Here's how the part is built. I have some questions about the finished solid (model axes, mm). A direction names the side the tool comes from. Coordinates: 2 decimals unless noted, no trailing zeros. Write each loop counter-clockwise with the first axis right and the second up, starting at its lowest first coordinate (ties: lowest second). Pieces come first, ordered by that corner, then holes. Notation, with made-up numbers: (34.25, -9) -> (50.25, -9) arc R22 cw to (50.25, 8) -> close; hole circle Ø3 at (57.25, 27). An arc over 180 degrees is marked (long way). Put each result on its own line as item: value.
Autodesk Inventor part; units mm, degrees
ref_plane "Work Plane1" through (0, -11, 0) normal (0, 1, 0) x (-1, 0, 0)
ref_plane "Work Plane2" through (9.5263, 5.5, -10) normal (0.866, 0.5, 0) x (-0.5, 0.866, 0)
ref_plane "Work Plane3" through (-9.5263, 5.5, -10) normal (-0.866, 0.5, 0) x (-0.5, -0.866, 0)
sketch "Sketch1" plane through (0, 0, 0) normal (0, 0, 1) x (1, 0, 0)
  circle A0 centre (0, 0) radius 35
  dimension "d0" = 70
extrude "Extrusion1" add sketch "Sketch1" along normal blind 7
sketch "Sketch2" plane through (0, 0, 7) normal (0, 0, 1) x (1, 0, 0)
  circle A0 centre (0, 0) radius 35
  circle A1 centre (0, 0) radius 23 construction
  line L0 (0, 0) -> (0, 23) construction
  point P0 (-16.2635, 16.2635)
  point P1 (-23, 0)
  point P2 (-16.2635, -16.2635)
  point P3 (0, -23)
  point P4 (16.2635, -16.2635)
  point P5 (23, 0)
  point P6 (16.2635, 16.2635)
  dimension "d3" = 46
  dimension "d6" = 360
hole "Hole1" at (0, 23, 7) at (-16.2635, 16.2635, 7) at (-23, 0, 7) at (-16.2635, -16.2635, 7) at (0, -23, 7) at (16.2635, -16.2635, 7) at (23, 0, 7) at (16.2635, 16.2635, 7) direction (0, 0, -1) diameter 15 depth 5
fillet "Fillet2" radius 1 1 edges at (-35, 0, 7)
sketch "Sketch12" plane through (0, 0, 0) normal (0, 0, -1) x (-1, 0, 0)
  circle A0 centre (0, 0) radius 35
  circle A1 centre (0, 0) radius 11
  dimension "d62" = 22
extrude "Extrusion4" add sketch "Sketch12" along normal blind 10 contours A1
sketch "Sketch13" plane through (0, 0, -10) normal (0, 0, -1) x (-1, 0, 0)
  point P0 (0, 0)
  point P1 (0, 0)
hole "Hole6" at (0, 0, -10) direction (0, 0, 1) diameter 8 end through all
sketch "Sketch14" plane through (0, 0, 7) normal (0, 0, 1) x (1, 0, 0)
  circle A0 centre (0, 0) radius 28 construction
  circle A1 centre (0, 0) radius 4
  circle A2 centre (16.2635, 16.2635) radius 7.5
  circle A3 centre (16.2635, -16.2635) radius 7.5
  circle A4 centre (-16.2635, -16.2635) radius 7.5
  circle A5 centre (-16.2635, 16.2635) radius 7.5
  circle A6 centre (0, 23) radius 7.5
  circle A7 centre (-23, 0) radius 7.5
  circle A8 centre (0, -23) radius 7.5
  circle A9 centre (23, 0) radius 7.5
  circle A10 centre (0, 0) radius 34
  circle A11 centre (0, 0) radius 4
  line L0 (0, 0) -> (16.2635, 16.2635)
  line L1 (0, 0) -> (10.7151, 25.8686)
  line L2 (25.8686, 10.7151) -> (0, 0)
  line L3 (16.2635, -16.2635) -> (-16.2635, 16.2635)
  point P0 (-25.8686, -10.7151)
  point P1 (-10.7151, -25.8686)
  dimension "d72" = 56
  dimension "d73" = 22.5
  dimension "d74" = 22.5
hole "Hole7" at (25.8686, 10.7151, 7) at (10.7151, 25.8686, 7) at (-10.7151, -25.8686, 7) at (-25.8686, -10.7151, 7) direction (0, 0, -1) diameter 4.134 end through all
ref_plane "Work Plane1" through (0, -11, 0) normal (0, 1, 0) x (-1, 0, 0)
sketch "Sketch15" plane through (0, -11, 0) normal (0, 1, 0) x (-1, 0, 0)
  line L0 (-11, -10) -> (11, -10)
  line L1 (11, 0) -> (-11, 0)
  line L2 (-11, 0) -> (-11, -10)
  line L3 (11, 0) -> (-11, 0)
  line L4 (-11, 0) -> (-11, -3)
  line L5 (-11, -3) -> (11, -3)
  line L6 (11, -3) -> (11, 0)
  point P0 (0, 0)
  point P1 (0, -5)
  dimension "d82" = 3
  dimension "d83" = 11
  dimension "d84" = 5
hole "Hole8" at (0, -11, -5) direction (0, 1, 0) diameter 3.242 depth 11.05 tip angle 118
sketch "Sketch16" plane through (0, 0, -10) normal (0, 0, -1) x (-1, 0, 0)
  circle A0 centre (0, 0) radius 4
  circle A1 centre (0, 0) radius 11
  line L0 (0, 0) -> (0, -11)
  circle A2 centre (0, 0) radius 11
  line L1 (0, 0) -> (-9.5263, 5.5)
  line L2 (0, 0) -> (9.5263, 5.5)
  dimension "d92" = 120
  dimension "d93" = 120
ref_plane "Work Plane2" through (9.5263, 5.5, -10) normal (0.866, 0.5, 0) x (-0.5, 0.866, 0)
ref_plane "Work Plane3" through (-9.5263, 5.5, -10) normal (-0.866, 0.5, 0) x (-0.5, -0.866, 0)
sketch "Sketch17" plane through (9.5263, 5.5, -10) normal (0.866, 0.5, 0) x (-0.5, 0.866, 0)
  line L0 (35, 10) -> (-35, 10)
  line L1 (35, 16) -> (-35, 16)
  line L2 (-11, 0) -> (11, 0)
  line L3 (11, 10) -> (11, 0)
  line L4 (-11, 10) -> (-11, 0)
  point P0 (0, 10)
  point P1 (0, 5)
  dimension "d94" = 11
  dimension "d95" = 5
hole "Hole9" at (9.5263, 5.5, -5) direction (-0.866, -0.5, 0) diameter 3.242 depth 11.05 tip angle 118
sketch "Sketch18" plane through (-9.5263, 5.5, -10) normal (-0.866, 0.5, 0) x (-0.5, -0.866, 0)
  line L0 (11, 10) -> (11, 0)
  line L1 (35, 10) -> (-35, 10)
  line L2 (-11, 0) -> (11, 0)
  line L3 (-11, 10) -> (-11, 0)
  point P0 (0, 10)
  point P1 (0, 5)
  dimension "d103" = 5
  dimension "d104" = 11
hole "Hole10" at (-9.5263, 5.5, -5) direction (0.866, -0.5, 0) diameter 3.242 depth 11.05 tip angle 118
properties part number "P003" material "Aluminum 6061"
Item 1: For P1, Ø13.5, axis at x = -23, y = 0, coming from the +Z side; P2, Ø8, axis at y = 10, z = -5.5, coming from the -X side; P3, Ø4, axis at y = -7, z = -1.5, coming from the +X side, each with a flat end and sliding along its axis, tell me the tip position at first contact or that it passes through.
Output:
P1: stops at z = 2
P2: stops at x = -9.14
P3: stops at x = 34.54
Item 2: Imagine slicing it at D-D on z = -5. Write out the boundary of the cut face in (x, y), then the cut area to 3 significant figures.
Output:
outline: (-10.23, 4.04) arc R11 ccw to (-1.62, -10.88) -> (-1.62, -3.66) arc R4 cw to (-3.98, 0.42) -> close; (-8.61, 6.84) -> (-2.36, 3.23) arc R4 cw to (2.36, 3.23) -> (8.61, 6.84) arc R11 ccw to start; (1.62, -10.88) arc R11 ccw to (10.23, 4.04) -> (3.98, 0.42) arc R4 cw to (1.62, -3.66) -> close
area: 261 mm²
Item 3: Imagine slicing it at B-B on z = 4.75. State how many separate pieces and enclosed holes the cut face has, then the cut area to 3 significant figures.
Output:
separate pieces: 1
enclosed holes: 13
area: 2,330 mm²
Item 4: If we mould it in two halves opening along Z, with no side actions, what happens to faces 1 (the flat face through (-23, 0, 2)), 2 (the cylindrical face through (-8.7, -25.4, 3.5)), 3 (the cylindrical face through (0.986, -7.277, -3.714)), 4 (the flat face through (0, -5, -10))? For each: released by +Z, released by -Z, zero draft, split by the parting line, or undercut.
Output:
face 1: released by +Z
face 2: zero draft
face 3: undercut
face 4: released by -Z
Item 5: Which directions (+Z, -Z, +X, -X, +Y, -Y) give clear straight access to the entire face, cutting with the end or side of a thin tool? Please do faces 5 (the cylindrical face through (-23.7, -15.3, 4.5)), 6 (the flat face through (-8, 8, 0)), 7 (the cylindrical face through (-6.545, 3.217, -3.454)).
Output:
face 5: +Z
face 6: -Z
face 7: none
Item 6: Please list where these lines run through material, in increasing order: line 1 along Y through (x, z) = (0, 4.95); line 2 along Y through (x, z) = (-26, 3.5); line 3 along Z through (x, y) = (0, -9). Write a range as from..to.
Output:
line 1: y = -35..-30.5, -15.5..-4, 4..15.5, 30.5..35
line 2: y = -23.43..-12.78, -8.65..-6.87, 6.87..23.43
line 3: z = -10..-6.62, -3.38..7
Item 7: Imagine slicing it at C-C on z = -1. Write out the boundary of the cut face in (x, y), then the cut area to 3 significant figures.
Output:
outline: circle Ø22 at (0, 0); hole circle Ø8 at (0, 0)
area: 330 mm²
Item 8: Imagine slicing it at A-A on x = 0. Write out the boundary of the cut face in (y, z), then the cut area to 3 significant figures.
Output:
outline: (-35, 0) -> (-11, 0) -> (-11, -3.38) -> (-4, -3.38) -> (-4, 7) -> (-15.5, 7) -> (-15.5, 2) -> (-30.5, 2) -> (-30.5, 7) -> (-34, 7) arc R1 ccw to (-35, 6) -> close; (-11, -10) -> (-4, -10) -> (-4, -6.62) -> (-11, -6.62) -> close; (4, -10) -> (11, -10) -> (11, 0) -> (35, 0) -> (35, 6) arc R1 ccw to (34, 7) -> (30.5, 7) -> (30.5, 2) -> (15.5, 2) -> (15.5, 7) -> (4, 7) -> close
area: 401 mm²
